Design review of the part built by this model. Coordinates are the model's own, in mm. A direction names the side the tool comes from. Coordinates: 2 decimals unless noted, no trailing zeros. Loops run counter-clockwise (first coordinate to the right, second up) from the corner with the lowest first, then second, coordinate; pieces in that order, holes last. Notation, with made-up numbers: M -10,-9.5 L 43,-9.5 A22 ccw 43,25.5 Z; hole C 88.5,74 d5. An arc over 180 degrees is marked long. One line per item, written item: value.
```python
from build123d import *

# Parameters (mm, degrees)
SKETCH4_R          = 14
CUT_EXTRUDE1_DEPTH = 8
SKETCH5_R          = 12.5
CUT_EXTRUDE4_DEPTH = 8.1
SKETCH7_R          = 2.5
CUT_EXTRUDE5_DEPTH = 3


with BuildPart() as part:
    # Sketch2 → Revolve4 (revolve)
    with BuildSketch(Plane(origin=(0, 0, 0), x_dir=(1, 0, 0), z_dir=(0, 1, 0)), mode=Mode.PRIVATE) as revolve4_sk:
        Polygon((0, 0), (-30, 0), (-30, -7), (-17, -7), (-17, -12), (0, -12), align=None)
    revolve(revolve4_sk.sketch.rotate(Axis((0, 0, 12), (0, 0, -1)), 180), axis=Axis((0, 0, 12), (0, 0, -1)))

    # Sketch4 → Cut-Extrude1 (cut)
    with BuildSketch(Plane.XY.offset(12)):
        Circle(SKETCH4_R)
    extrude(amount=-CUT_EXTRUDE1_DEPTH, mode=Mode.SUBTRACT)

    # Sketch5 → Cut-Extrude4 (cut)
    with BuildSketch(Plane(origin=(0, 0, 0), x_dir=(-1, 0, 0), z_dir=(0, 0, -1))):
        Circle(SKETCH5_R)
    extrude(amount=-CUT_EXTRUDE4_DEPTH, mode=Mode.SUBTRACT)

    # Sketch7 → Cut-Extrude5 (cut)
    with BuildSketch(Plane(origin=(0, 0, 0), x_dir=(-1, 0, 0), z_dir=(0, 0, -1))):
        with Locations((0, 18)):
            Circle(SKETCH7_R)
        with Locations((15.588457268, 9)):
            Circle(SKETCH7_R)
        with Locations((15.588457268, -9)):
            Circle(SKETCH7_R)
        with Locations((0, -18)):
            Circle(SKETCH7_R)
        with Locations((-15.588457268, -9)):
            Circle(SKETCH7_R)
        with Locations((-15.588457268, 9)):
            Circle(SKETCH7_R)
    extrude(amount=-CUT_EXTRUDE5_DEPTH, mode=Mode.SUBTRACT)


solid = part.part
```
(1) We need section B-B on x = 0. State the section outline as (y, z) points.
Reply:
outline: M -30,0 L -20.5,0 L -20.5,3 L -15.5,3 L -15.5,0 L -12.5,0 L -12.5,4 L -14,4 L -14,12 L -17,12 L -17,7 L -30,7 Z; M 12.5,0 L 15.5,0 L 15.5,3 L 20.5,3 L 20.5,0 L 30,0 L 30,7 L 17,7 L 17,12 L 14,12 L 14,4 L 12.5,4 Z
(2) Mouldability with a two-part tool opening along X and no side actions: class faces 1 (the flat face through (0, 18, 3)), 2 (the flat face through (-6, -13, 12)), 3 (the cylindrical face through (16.128, -25.296, 3.549)), 4 (the cylindrical face through (-11.923, 3.755, 1.972)) as released by +X, released by -X, zero draft, split by the parting line, or undercut.
Reply:
face 1: undercut
face 2: zero draft
face 3: split by the parting line
face 4: undercut
(3) Insertion check: pin 1 (1 mm diameter, centred on x = 12.5, z = 6.5, fed in from -Y); pin 2 (14 mm diameter, centred on x = -1, y = 3.5, fed in from +Z) (3 decimals); pin 3 (4 mm diameter, centred on x = -21, z = 6.5, fed in from -Y); pin 4 (5 mm diameter, centred on y = 18, z = 5.5, fed in from -X). Each pin has a flat end and moves straight along its axis. Give the tip position at first contact, or say it passes through.
Reply:
pin 1: stops at y = -27.5
pin 2: passes through
pin 3: stops at y = -23.22
pin 4: stops at x = -25.69
(4) Tool access review of faces 5 (the cylindrical face through (12.932, -5.362, 8.056)), 6 (the cylindrical face through (-2.385, -17.249, 1.479)): name each direction out of +Z, -Z, +X, -X, +Y, -Y from which nothing blocks a thin tool from reaching the whole face with its end or side.
Reply:
face 5: +Z
face 6: -Z
(5) We need section C-C on z = 2. State the section outline as (x, y) points, then the cut area to 3 significant figures.
Reply:
outline: C 0,0 d60; hole C -15.59,-9 d5; hole C -15.59,9 d5; hole C 0,0 d25; hole C 0,-18 d5; hole C 0,18 d5; hole C 15.59,-9 d5; hole C 15.59,9 d5
area: 2,220 mm2
(6) We need section D-D on y = -18. State the section outline as (x, z) points.
Reply:
outline: M -24,0 L -2.5,0 L -2.5,3 L 2.5,3 L 2.5,0 L 24,0 L 24,7 L -24,7 Z
(7) We need section A-A on y = 0. State the section outline as (x, z) points.
Reply:
outline: M -30,0 L -12.5,0 L -12.5,4 L -14,4 L -14,12 L -17,12 L -17,7 L -30,7 Z; M 12.5,0 L 30,0 L 30,7 L 17,7 L 17,12 L 14,12 L 14,4 L 12.5,4 Z
(8) To check wall thickness, follow line 1 along Y through (x, z) = (0, 2.25); line 2 along Y through (x, z) = (0, 6); line 3 along X through (y, z) = (0.5, 8.25). State the ranges of each line that lie inside material, in increasing order. Write a range as [from, to].
Reply:
line 1: y = [-30, -20.5], [-15.5, -12.5], [12.5, 15.5], [20.5, 30]
line 2: y = [-30, -14], [14, 30]
line 3: x = [-16.99, -13.99], [13.99, 16.99]
